Study the drawing (mm; zero at the part's minimum x, y, z) and answer. Give positions to 0.01 mm unless a question says otherwise; leave off trailing zeros. Write each loop counter-clockwise with the first axis right and the second up, starting at its lowest first coordinate (ties: lowest second). Pieces come first, ordered by that corner, then holes. Notation, with made-up numbers: (-40, 33) - (-5, 33) arc R33 cw to (-5, 70) - close; hole circle Ø2 at (40, 27.5). An arc over 180 degrees is marked (long way). Write each question's results on one line, items separated by ' | '. Start each with the question number.
Q1. Section A-A (x = 8.5) is taken. Determine the outline of the cut face in (y, z), plus the area to 3 significant figures.
Q2. Section D-D (x = 48.75) is taken. Determine the outline of the cut face in (y, z).
Q3. Flat-ended cylindrical pins translate along their axes: pin 1 Ø8 at (x, z) = (8.5, 8.5) entering from +Y; pin 2 Ø4.5 at (x, z) = (48.75, 8.5) entering from +Y. Find the tip coordinate at first contact, or state that the pin passes through.
Q4. Find the intervals of material crossed by probe 1 along X at (y, z) = (2.6, 189.5); probe 2 along X at (y, z) = (2.6, 99), in increasing order.
Q5. Section C-C (z = 189.5) is taken. Determine the outline of the cut face in (x, y), plus the area to 3 significant figures.
Q6. Section B-B (z = 48.75) is taken. Determine the outline of the cut face in (x, y).
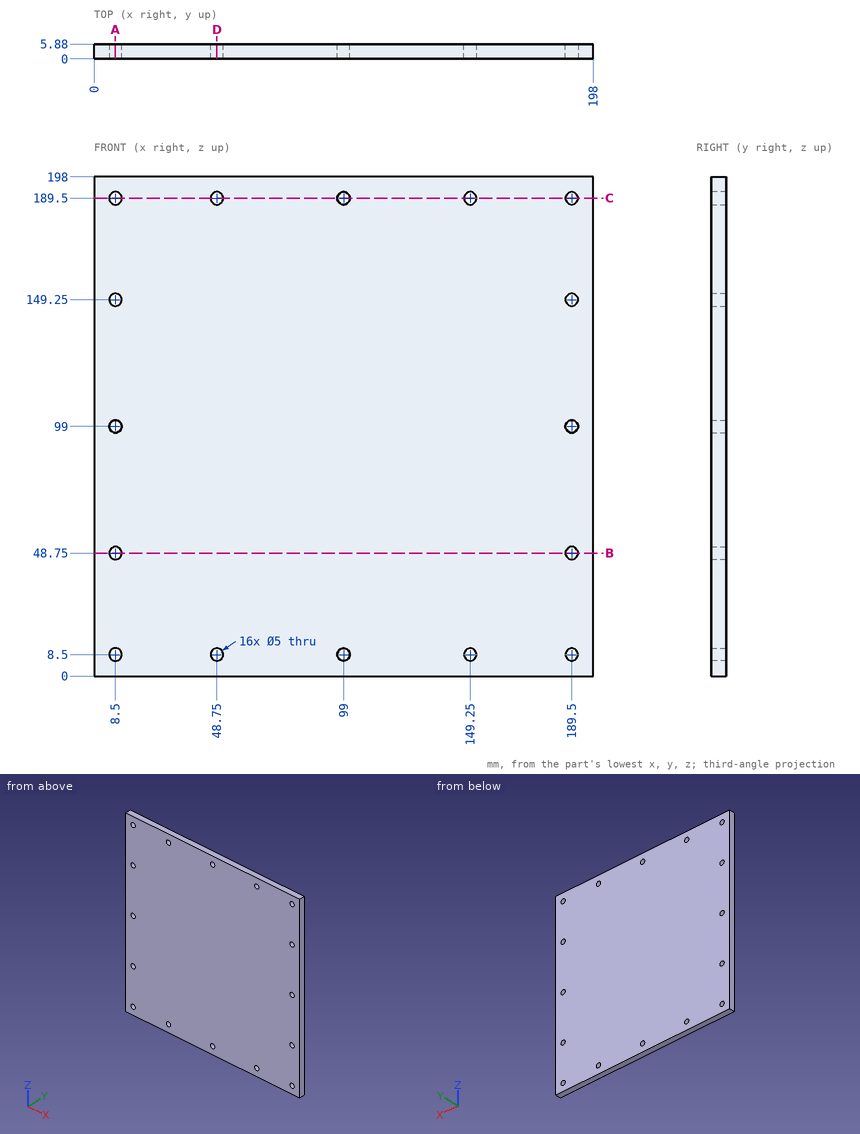
Answers below:
1) outline: (0, 0) - (5.88, 0) - (5.88, 6) - (0, 6) - close; (0, 11) - (5.88, 11) - (5.88, 46.25) - (0, 46.25) - close; (0, 51.25) - (5.88, 51.25) - (5.88, 96.5) - (0, 96.5) - close; (0, 101.5) - (5.88, 101.5) - (5.88, 146.75) - (0, 146.75) - close; (0, 151.75) - (5.88, 151.75) - (5.88, 187) - (0, 187) - close; (0, 192) - (5.88, 192) - (5.88, 198) - (0, 198) - close | area: 1,020 mm2
2) outline: (0, 0) - (5.88, 0) - (5.88, 6) - (0, 6) - close; (0, 11) - (5.88, 11) - (5.88, 187) - (0, 187) - close; (0, 192) - (5.88, 192) - (5.88, 198) - (0, 198) - close
3) pin 1: stops at y = 5.88 | pin 2: passes through
4) probe 1: x = 0 to 6, 11 to 46.25, 51.25 to 96.5, 101.5 to 146.75, 151.75 to 187, 192 to 198 | probe 2: x = 0 to 6, 11 to 187, 192 to 198
5) outline: (0, 0) - (6, 0) - (6, 5.88) - (0, 5.88) - close; (11, 0) - (46.25, 0) - (46.25, 5.88) - (11, 5.88) - close; (51.25, 0) - (96.5, 0) - (96.5, 5.88) - (51.25, 5.88) - close; (101.5, 0) - (146.75, 0) - (146.75, 5.88) - (101.5, 5.88) - close; (151.75, 0) - (187, 0) - (187, 5.88) - (151.75, 5.88) - close; (192, 0) - (198, 0) - (198, 5.88) - (192, 5.88) - close | area: 1,020 mm2
6) outline: (0, 0) - (6, 0) - (6, 5.88) - (0, 5.88) - close; (11, 0) - (187, 0) - (187, 5.88) - (11, 5.88) - close; (192, 0) - (198, 0) - (198, 5.88) - (192, 5.88) - close
